```python
from build123d import *

# Parameters (mm, degrees)
PRISM_DEPTH       = 70
SKETCH001_R       = 10
EXTRUDE001_DEPTH  = 25
CYLINDER002_R     = 20
CYLINDER002_DEPTH = 7
PRISM001_DEPTH    = 12
CYLINDER001_R     = 45
CYLINDER001_DEPTH = 25
FILLET003_R       = 3
CYLINDER003_R     = 15
CYLINDER003_DEPTH = 150
EXTRUDE_DEPTH     = 15
FILLET_R          = 5
FILLET001_R       = 2
CYLINDER_R        = 40
CYLINDER_DEPTH    = 200
FILLET002_R       = 20


with BuildPart() as prisma:
    # Prism → Prism (new body)
    with BuildSketch(Plane(origin=(50, 0, 0), x_dir=(1, 0, 0), z_dir=(0, 0, 1))):
        Polygon((10, 0), (5, 8.660254), (-5, 8.660254), (-10, 0), (-5, -8.660254), (5, -8.660254), align=None)
    extrude(amount=PRISM_DEPTH)


with BuildPart() as fusion001:
    # Sketch001 → Extrude001 (new body)
    with BuildSketch(Plane.XY):
        with Locations((50, 0)):
            Circle(SKETCH001_R)
    extrude(amount=EXTRUDE001_DEPTH)

    # Fusion001: union Prisma
    add(prisma.part)


with BuildPart() as cilindro002:
    # Cylinder002 → Cylinder002 (new body)
    with BuildSketch(Plane(origin=(-5, 0, 200), x_dir=(1, 0, 0), z_dir=(0, 0, 1))):
        Circle(CYLINDER002_R)
    extrude(amount=CYLINDER002_DEPTH)


with BuildPart() as fusion004:
    # Prism001 → Prism001 (new body)
    with BuildSketch(Plane(origin=(-5, 0, 200), x_dir=(1, 0, 0), z_dir=(0, 0, 1))):
        Polygon((19, 0), (9.5, 16.454483), (-9.5, 16.454483), (-19, 0), (-9.5, -16.454483), (9.5, -16.454483), align=None)
    extrude(amount=PRISM001_DEPTH)

    # Fusion: union Cilindro002
    add(cilindro002.part)

    # Fusion004: union Fusion001
    add(fusion001.part)


with BuildPart() as fillet003:
    # Cylinder001 → Cylinder001 (new body)
    with BuildSketch(Plane(origin=(-5, 0, 0), x_dir=(1, 0, 0), z_dir=(0, 0, 1))):
        Circle(CYLINDER001_R)
    extrude(amount=CYLINDER001_DEPTH)

    # Fillet003
    fillet003_edges = [fillet003.edges().sort_by_distance(p)[0] for p in [
        (-50, 0, 25),
    ]]
    fillet(fillet003_edges, radius=FILLET003_R)


with BuildPart() as fusion003:
    # Cylinder003 → Cylinder003 (new body)
    with BuildSketch(Plane(origin=(-5, 0, 90), x_dir=(1, 0, 0), z_dir=(0, 0, 1))):
        Circle(CYLINDER003_R)
    extrude(amount=CYLINDER003_DEPTH)

    # Fusion003: union Fillet003
    add(fillet003.part)


with BuildPart() as fillet001:
    # Sketch → Extrude (new body)
    with BuildSketch(Plane.XY):
        Polygon((-50, 50), (-50, -50), (50, -50), (50, -15), (60, -15), (60, 15), (50, 15), (50, 50), align=None)
    extrude(amount=EXTRUDE_DEPTH)

    # Fillet
    fillet_edges = [fillet001.edges().sort_by_distance(p)[0] for p in [
        (-50, 50, 7.5),
        (-50, -50, 7.5),
        (50, -50, 7.5),
        (50, -15, 7.5),
        (50, 15, 7.5),
        (50, 50, 7.5),
    ]]
    fillet(fillet_edges, radius=FILLET_R)

    # Fillet001
    fillet001_edges = [fillet001.edges().sort_by_distance(p)[0] for p in [
        (-50, 0, 15),
        (-48.535534, 48.535534, 15),
        (-48.535534, -48.535534, 15),
        (0, 50, 15),
        (0, -50, 15),
        (48.535534, 48.535534, 15),
        (48.535534, -48.535534, 15),
        (50, 32.5, 15),
        (50, -32.5, 15),
        (51.464466, 16.464466, 15),
        (51.464466, -16.464466, 15),
        (57.5, 15, 15),
        (57.5, -15, 15),
        (60, 0, 15),
    ]]
    fillet(fillet001_edges, radius=FILLET001_R)


with BuildPart() as obj1:
    # Cylinder → Cylinder (new body)
    with BuildSketch(Plane(origin=(-5, 0, 0), x_dir=(1, 0, 0), z_dir=(0, 0, 1))):
        Circle(CYLINDER_R)
    extrude(amount=CYLINDER_DEPTH)

    # Fillet002
    fillet002_edges = [obj1.edges().sort_by_distance(p)[0] for p in [
        (-45, 0, 200),
    ]]
    fillet(fillet002_edges, radius=FILLET002_R)

    # Fusion002: union Fillet001
    add(fillet001.part)

    # Fusion005: union Fusion004, Fusion003
    add(fusion004.part)
    add(fusion003.part)


solid = obj1.part
```
Read the model definition and answer for the solid it produces. Units are mm, in the model's axes. A direction names the side the tool comes from. Give positions to 0.01 mm unless a question says otherwise; leave off trailing zeros. Loops run counter-clockwise (first coordinate to the right, second up) from the corner with the lowest first, then second, coordinate; pieces in that order, holes last.
Item 1: Each of these flat-tipped pins is pushed along its axis until it touches: pin 1 Ø24 at (x, y) = (-15, 35.5) entering from +Z; pin 2 Ø10.5 at (y, z) = (-38, 5) entering from +X; pin 3 Ø8 at (x, z) = (11, 31.5) entering from -Y. Where does it stop, or does it pass through?
Item 2: The part is cut by section B-B (z = 104.5). Write down the section's boundary in (x, y), and give its area (3 significant figures).
Item 3: Find the intervals of material crossed by line 1 along Z through (x, y) = (43, -43); line 2 along Z through (x, y) = (46.5, 9); line 3 along Y through (x, z) = (-3, 105.5), in increasing order.
Item 4: For faces 5 (the flat face through (17, 40, 15)), 6 (the flat face through (32.1, -15.4, 25)), 7 (the flat face through (57.535, 4.27, 47.185)), determine the directions among +Z, -Z, +X, -X, +Y, -Y from which every point of the face is accessible in a straight line to the end or side of a thin tool.
Item 5: The mould has two halves that part along X. Classify faces 1 (the flat face through (42, 5, 25)), 2 (the flat face through (42.465, -4.27, 47.185)), 3 (the cylindrical face through (-21, -12, 203)), 4 (the cylindrical face through (51, -17, 7)): released by +X, released by -X, zero draft, split by the parting line, or undercut.
Item 6: The part is cut by section A-A (z = 202.5). Write down the section's boundary in (x, y), and give its area (3 significant figures).
Taken from the geometry:
1. pin 1: stops at z = 199.4
1. pin 2: stops at x = 50
1. pin 3: stops at y = -38.16
2. outline: circle Ø80 at (-5, 0)
2. area: 5,030 mm2
3. line 1: z = 0 to 15
3. line 2: z = 0 to 25
3. line 3: y = -39.95 to 39.95
4. face 5: +Z, +Y
4. face 6: +Z
4. face 7: +Z, +X, +Y
5. face 1: undercut
5. face 2: undercut
5. face 3: split by the parting line
5. face 4: released by +X
6. outline: circle Ø40 at (-5, 0)
6. area: 1,260 mm2
